Autodesk Inventor part; units mm, degrees
ref_plane "YZ Plane" through (0, 0, 0) normal (1, 0, 0) x (0, 1, 0)
ref_plane "XZ Plane" through (0, 0, 0) normal (0, 1, 0) x (-1, 0, 0)
ref_plane "XY Plane" through (0, 0, 0) normal (0, 0, 1) x (1, 0, 0)
sketch "Sketch1" plane through (0, 0, 0) normal (0, 0, 1) x (1, 0, 0)
  circle A0 centre (0, 0) radius 26.1874
  circle A1 centre (0, 0) radius 23.6474
  dimension "d0" = 52.3748
  dimension "d1" = 2.54
extrude "Extrusion1" add sketch "Sketch1" along normal mid plane 145.288
sketch "Sketch2" plane through (0, 0, 0) normal (1, 0, 0) x (0, 1, 0)
  line L0 (-26.1874, 72.644) -> (26.1874, 72.644)
  line L1 (-23.6474, 72.644) -> (23.6474, 72.644)
  line L2 (26.1874, 72.644) -> (25.4, 72.644)
  line L3 (25.4, 72.644) -> (25.4, 71.0565)
  line L4 (25.4, 71.0565) -> (26.1874, 71.0565)
  line L5 (26.1874, 71.0565) -> (26.1874, 72.644)
  line L6 (0, -14.5288) -> (0, 87.1728)
  point P0 (0, 0)
  dimension "d4" = 1.5875
  dimension "d5" = 0.7874
revolve "Revolution1" cut sketch "Sketch2" angle 360 about axis through (0, 0, -10) along (0, 0, 1)
mirror "Mirror1" about plane through (0, 0, 0) normal (0, 0, 1) of "Revolution1"
properties material "Stainless Steel"
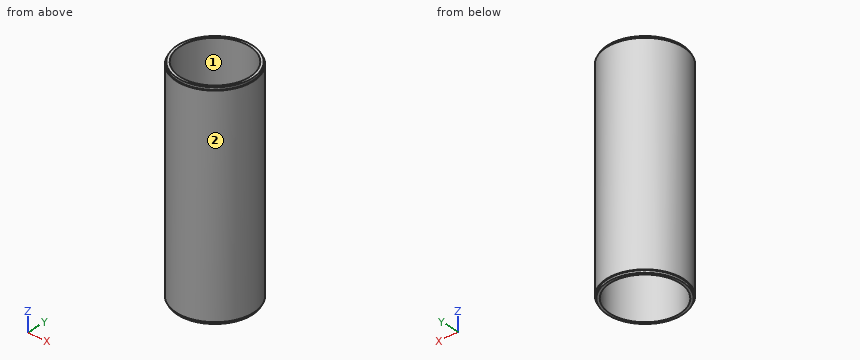
Can you work these out from the model? Positions are in its coordinate system, mm. Face numbers are marked on the shaded views. Round coordinates to 2 decimals unless told otherwise and drop trailing zeros. Write each loop counter-clockwise with the first axis right and the second up, starting at its lowest first coordinate (ties: lowest second). Pieces come first, ordered by that corner, then holes. Notation, with made-up numbers: M 59.5,-9.5 L 73.5,-9.5 A5 ccw 73.5,-1.5 Z; hole C 40,58 d5. An arc over 180 degrees is marked long. Use a Markdown table: item, result.
Item 1: For pin 1 Ø8 at (y, z) = (12.5, 48) entering from +X; pin 2 Ø3 at (x, z) = (-13.5, -20.5) entering from +Y; pin 3 Ø1 at (y, z) = (4.5, 16) entering from +X, each with a flat end and sliding along its axis, tell me the tip position at first contact or that it passes through.
Found:
| item | result |
|---|---|
| pin 1 | stops at x = 24.77 |
| pin 2 | stops at y = 23.28 |
| pin 3 | stops at x = 25.88 |
Item 2: I want a section at C-C (z = -40). List the corners of the cut face in (x, y) for me, and give its area (3 significant figures).
Found:
| item | result |
|---|---|
| outline | C 0,0 d52.37; hole C 0,0 d47.29 |
| area | 398 mm2 |
Item 3: If I drill on line 1 along Y through (x, z) = (0, 17.5); line 2 along X through (y, z) = (-20, 9); line 3 along Y through (x, z) = (9, -51.5), over which ranges is the centre line in solid material (lowest first)? Write a range as [from, to].
Found:
| item | result |
|---|---|
| line 1 | y = [-26.19, -23.65], [23.65, 26.19] |
| line 2 | x = [-16.91, -12.62], [12.62, 16.91] |
| line 3 | y = [-24.59, -21.87], [21.87, 24.59] |
Item 4: I want a section at A-A (y = 0). List the corners of the cut face in (x, z) for me, and give its area (3 significant figures).
Found:
| item | result |
|---|---|
| outline | M -26.19,-71.06 L -25.4,-71.06 L -25.4,-72.64 L -23.65,-72.64 L -23.65,72.64 L -25.4,72.64 L -25.4,71.06 L -26.19,71.06 Z; M 23.65,-72.64 L 25.4,-72.64 L 25.4,-71.06 L 26.19,-71.06 L 26.19,71.06 L 25.4,71.06 L 25.4,72.64 L 23.65,72.64 Z |
| area | 733 mm2 |
Item 5: We'd pull the mould along Y, two halves only. Please class the marked faces 1 and 2: released by +Y, released by -Y, zero draft, split by the parting line, or undercut.
Found:
| item | result |
|---|---|
| face 1 | undercut |
| face 2 | split by the parting line |
